Could you check a few things on this model? Use its own coordinates, in mm. A direction names the side the tool comes from. Coordinates: 2 decimals unless noted, no trailing zeros. Loops run counter-clockwise (first coordinate to the right, second up) from the corner with the lowest first, then second, coordinate; pieces in that order, holes last.
1) Thinking about a two-plate mould opening in X: for faces 4 (the face through (-29.91, -18.08, 22.74)), 5 (the face through (-6.073, -7.364, 22.736)), 6 (the face through (-53.914, -13, 35)), 7 (the face through (-37, 0, 27)), which applies, released by +X, released by -X, zero draft, split by the parting line, or undercut?
2) For faces 1 (the face through (-19, -13, 29.645)), 2 (the face through (-47.47, -2.19, 60.69)), 3 (the face through (-47, -6.486, 59)), which set-ups out of +Z, -Z, +X, -X, +Y, -Y let a thin tool reach every point of the face, with its end or its side?
3) Imagine slicing it at D-D on x = -25. Please give me the cut outline in (y, z).
4) Will these pins go through, and if not, where does the flat tip stop? P1, Ø12.5, axis at y = -7.5, z = 42, coming from the +X side; P2, Ø11.5, axis at x = -9.49, y = -12.72, coming from the -Z side; P3, Ø12, axis at y = -22.5, z = 28, coming from the +X side.
5) Imagine slicing it at C-C on x = -47. Please give me the cut outline in (y, z).
6) If I drill on line 1 along X through (y, z) = (-11, 23); line 2 along X through (y, z) = (-8.5, 27); line 3 along Z through (x, y) = (-1.5, -12.25), over which ranges is the centre line in solid material (lowest first)?
7) Imagine slicing it at A-A on z = 61.5. Please give me the cut outline in (x, y).
8) Imagine slicing it at B-B on y = -10.5. Please give me the cut outline in (x, z).
```python
from build123d import *

# Parameters (mm, degrees)
F1_DEPTH = 25.4
F3_DEPTH = 12.701
F5_DEPTH = 14.014792
F6_R     = 6.35
F7_DEPTH = 14.014792
F9_DEPTH = 12.701


with BuildPart() as f1:
    # F0 (on Front) → F1 (new body)
    with BuildSketch(Plane.XZ):
        Polygon((-41.213709, 66.43077), (-53.913709, 66.43077), (-53.913709, 15.63077), (3.236291, 15.63077), (3.236291, 29.644562), (-41.213709, 29.644562), align=None)
    extrude(amount=F1_DEPTH)

    # F2 (on face) → F3 (cut, through all)
    with BuildSketch(Plane.YZ.offset(-41.213709)):
        with BuildLine():
            ThreePointArc((-25.4, 56.502793), (-12.139061, 66.23636), (0, 55.135097))
            Line((0, 55.135097), (0, 66.43077))
            Line((0, 66.43077), (-25.4, 66.43077))
            Line((-25.4, 66.43077), (-25.4, 56.502793))
        make_face()
    extrude(amount=-F3_DEPTH, mode=Mode.SUBTRACT)

    # F4 (on face) → F5 (cut, through all)
    with BuildSketch(Plane.XY.offset(29.644562)):
        with BuildLine():
            ThreePointArc((-9.146443, 0), (-0.370686, -3.842993), (3.236291, -12.718364))
            Line((3.236291, -12.718364), (3.236291, 0))
            Line((3.236291, 0), (-9.146443, 0))
        make_face()
        with BuildLine():
            ThreePointArc((3.236291, -12.718364), (-0.135122, -21.345181), (-8.462597, -25.4))
            Line((-8.462597, -25.4), (3.236291, -25.4))
            Line((3.236291, -25.4), (3.236291, -12.718364))
        make_face()
    extrude(amount=-F5_DEPTH, mode=Mode.SUBTRACT)

    # F6 (on face) → F7 (cut, through all)
    with BuildSketch(Plane.XY.offset(29.644562)):
        with Locations((-28.536622, -11.881827)):
            Circle(F6_R)
        with Locations((-9.486622, -12.718364)):
            Circle(F6_R)
    extrude(amount=-F7_DEPTH, mode=Mode.SUBTRACT)

    # F8 (on face) → F9 (cut, through all)
    with BuildSketch(Plane.YZ.offset(-41.213709)):
        with BuildLine():
            ThreePointArc((-19.186374, 53.286288), (-12.836374, 59.636288), (-6.486374, 53.286288))
            Line((-6.486374, 53.286288), (-6.486374, 64.594166))
            ThreePointArc((-6.486374, 64.594166), (-12.836374, 66.25512), (-19.186374, 64.594166))
            Line((-19.186374, 64.594166), (-19.186374, 53.286288))
        make_face()
        with BuildLine():
            ThreePointArc((-19.186374, 53.286288), (-12.836374, 46.936288), (-6.486374, 53.286288))
            ThreePointArc((-6.486374, 53.286288), (-12.836374, 59.636288), (-19.186374, 53.286288))
        make_face()
    extrude(amount=-F9_DEPTH, mode=Mode.SUBTRACT)


solid = f1.part
```
Filled in:
1. face 4: undercut
1. face 5: undercut
1. face 6: released by -X
1. face 7: zero draft
2. face 1: +Z, +X, +Y, -Y
2. face 2: +Z, +X, -X, +Y
2. face 3: +Z, +X, -X
3. outline: (-25.4, 15.63) - (-17.16, 15.63) - (-17.16, 29.64) - (-25.4, 29.64) - close; (-6.61, 15.63) - (0, 15.63) - (0, 29.64) - (-6.61, 29.64) - close
4. P1: stops at x = -41.21
4. P2: passes through
4. P3: stops at x = 2.66
5. outline: (-25.4, 15.63) - (0, 15.63) - (0, 55.14) arc R12.97 ccw to (-6.49, 64.59) - (-6.49, 53.29) arc R6.35 cw to (-19.19, 53.29) - (-19.19, 64.59) arc R12.97 ccw to (-25.4, 56.5) - close
6. line 1: x = -53.91 to -34.83, -22.25 to -15.6, -3.37 to 3.12
6. line 2: x = -53.91 to -33.91, -23.16 to -14.23, -4.74 to 2.52
6. line 3: z = 15.63 to 29.64
7. outline: (-53.91, -22.87) - (-41.21, -22.87) - (-41.21, -19.19) - (-53.91, -19.19) - close; (-53.91, -6.49) - (-41.21, -6.49) - (-41.21, -2.8) - (-53.91, -2.8) - close
8. outline: (-53.91, 15.63) - (-34.73, 15.63) - (-34.73, 29.64) - (-41.21, 29.64) - (-41.21, 47.38) - (-53.91, 47.38) - close; (-22.34, 15.63) - (-15.44, 15.63) - (-15.44, 29.64) - (-22.34, 29.64) - close; (-3.54, 15.63) - (3.04, 15.63) - (3.04, 29.64) - (-3.54, 29.64) - close
